Here's the drawing with two shaded views (mm, measured from the low corner). I have some questions. Give positions to 0.01 mm unless a question says otherwise; leave off trailing zeros. Loops run counter-clockwise (first coordinate to the right, second up) from the corner with the lowest first, then second, coordinate; pieces in that order, holes last. Notation, with made-up numbers: (-36, 46.5) -> (-30, 46.5) arc R22 ccw to (-30, 84.5) -> close; hole circle Ø11 at (12.25, 62). An arc over 180 degrees is marked (long way). Write each question's results on one line, items separated by ' | '. Start each with the question number.
Q1. If we section it at A-A, the plane z = 28: List the corners of the cut face in (x, y) for me.
Q2. If we section it at B-B, the plane y = 0.5: Give the number of separate pieces and of enclosed holes in the cut face, plus the area to 3 significant figures.
Q3. If we section it at C-C, the plane z = 83: List the corners of the cut face in (x, y) for me.
Q4. Will these pins go through, and if not, where does the flat tip stop? P1, Ø4, axis at x = 78, z = 83, coming from the +Y side; P2, Ø1.9, axis at x = 79, z = 8, coming from the +Y side; P3, Ø0.9, axis at x = 13, y = 1.5, coming from the -Z side.
Q5. If I drill on line 1 along X through (y, z) = (1.2, 68); line 2 along X through (y, z) = (1.95, 83); line 3 along Z through (x, y) = (23, 1.3), over which ranges is the centre line in solid material (lowest first)?
Q6. If we section it at D-D, the plane x = 68: List the corners of the cut face in (y, z) for me, plus the area to 3 significant figures.
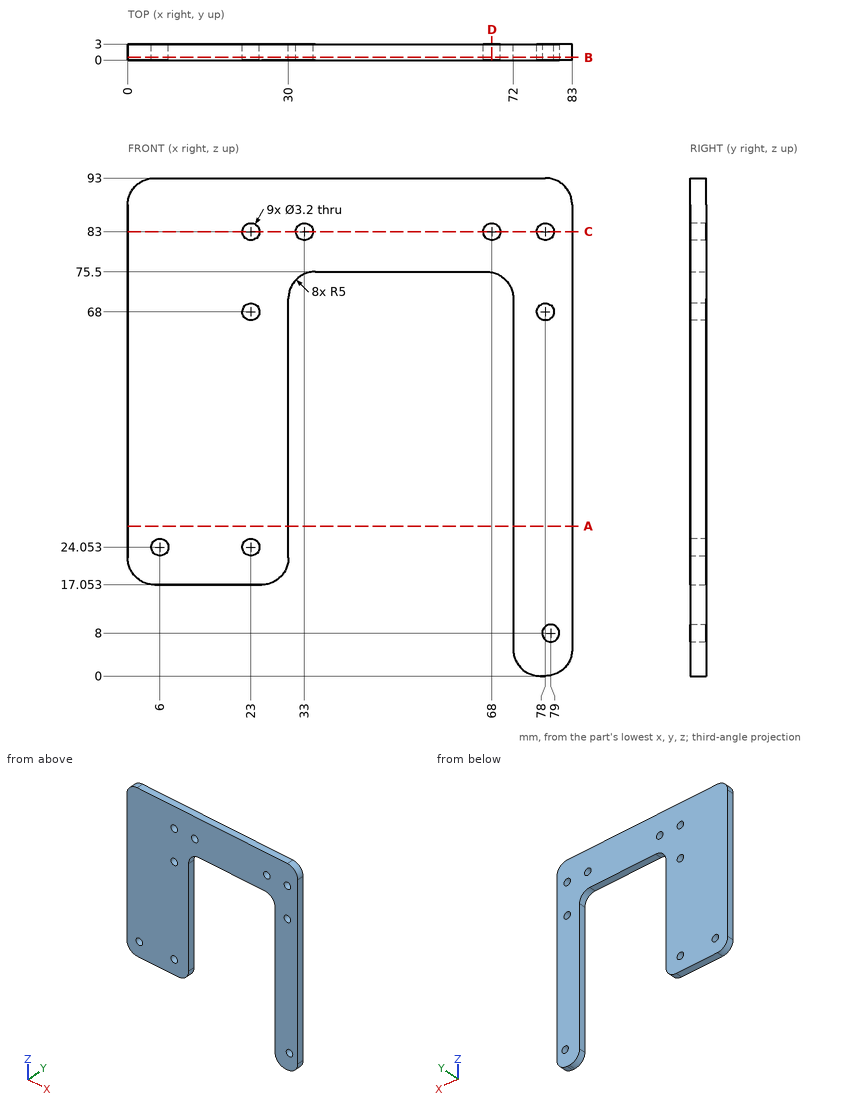
Final values:
1) outline: (0, 0) -> (30, 0) -> (30, 3) -> (0, 3) -> close; (72, 0) -> (83, 0) -> (83, 3) -> (72, 3) -> close
2) separate pieces: 1 | enclosed holes: 9 | area: 3,940 mm²
3) outline: (0, 0) -> (21.4, 0) -> (21.4, 3) -> (0, 3) -> close; (24.6, 0) -> (31.4, 0) -> (31.4, 3) -> (24.6, 3) -> close; (34.6, 0) -> (66.4, 0) -> (66.4, 3) -> (34.6, 3) -> close; (69.6, 0) -> (76.4, 0) -> (76.4, 3) -> (69.6, 3) -> close; (79.6, 0) -> (83, 0) -> (83, 3) -> (79.6, 3) -> close
4) P1: stops at y = 3 | P2: passes through | P3: stops at z = 17.05
5) line 1: x = 0 to 21.4, 24.6 to 30, 72 to 76.4, 79.6 to 83 | line 2: x = 0 to 21.4, 24.6 to 31.4, 34.6 to 66.4, 69.6 to 76.4, 79.6 to 83 | line 3: z = 17.05 to 22.45, 25.65 to 66.4, 69.6 to 81.4, 84.6 to 93
6) outline: (0, 75.4) -> (3, 75.4) -> (3, 81.4) -> (0, 81.4) -> close; (0, 84.6) -> (3, 84.6) -> (3, 93) -> (0, 93) -> close | area: 43.2 mm²
